The model under review builds one solid part; all positions refer to its coordinate system, in mm. Face numbers are marked on the shaded views. Give positions to 0.01 mm unless a question says otherwise; leave off trailing zeros. Loops run counter-clockwise (first coordinate to the right, second up) from the corner with the lowest first, then second, coordinate; pieces in that order, holes last. Notation, with made-up numbers: M 48,0.25 L 97,0.25 A25 ccw 97,35.25 Z; hole C -23.5,-16 d6. An arc over 180 degrees is marked long. One line per item, written item: value. Start each with the question number.
Q1. For pin 1 (3 mm diameter, centred on y = -3.11, z = 26.96, fed in from -X); pin 2 (1.5 mm diameter, centred on x = 0, y = 11, fed in from +Z); pin 3 (8 mm diameter, centred on x = -18.5, z = 3, fed in from -Y), all flat-tipped, find the tip position at first contact; note any pin that passes through.
Q2. Mouldability with a two-part tool opening along X and no side actions: class the marked faces 1, 2, 3 and 4 as released by +X, released by -X, zero draft, split by the parting line, or undercut.
Q3. We need section A-A on x = 0. Write out the cut boundary in (y, z).
Q4. We need section D-D on x = -11. Write out the cut boundary in (y, z).
Q5. To check wall thickness, follow line 1 along X through (y, z) = (-5, 15.5); line 2 along X through (y, z) = (0, -0.7); line 3 along Z through (x, y) = (-4, -10.5). State the ranges of each line that lie inside material, in increasing order. Write a range as from..to.
Q6. We need section B-B on z = 4.5. Write out the cut boundary in (x, y), plus the area to 3 significant figures.
Q7. We need section C-C on y = 11. Write out the cut boundary in (x, z), plus the area to 3 significant figures.
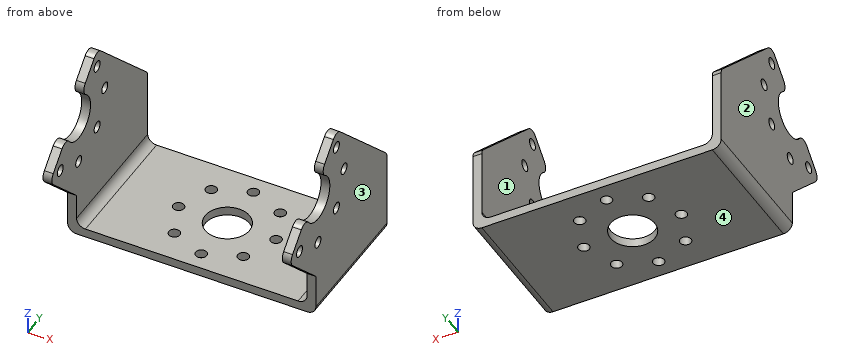
```python
from build123d import *

# Parameters (mm, degrees)
ESBO_O1_W                 = 56
ESBO_O1_H                 = 30
RESSALTO_EXTRUS_O1_DEPTH  = 2
RESSALTO_EXTRUS_O2_DEPTH  = 2
ESBO_O3_R                 = 5
CORTE_EXTRUS_O1_DEPTH     = 2
FILETE1_R                 = 2
ESBO_O4_R                 = 1.25
CORTE_EXTRUS_O2_DEPTH     = 2
PADR_OCIRCULAR1_COUNT     = 5
PADR_OCIRCULAR1_ANGLE     = 180
ESPELHAR3_COPY_1_SKETCH_R = 1.25
ESPELHAR3_COPY_1_DEPTH    = 2
ESPELHAR3_COPY_2_SKETCH_R = 1.25
ESPELHAR3_COPY_2_DEPTH    = 2
ESPELHAR3_COPY_3_SKETCH_R = 1.25
ESPELHAR3_COPY_3_DEPTH    = 2
ESPELHAR3_COPY_4_SKETCH_R = 1.25
ESPELHAR3_COPY_4_DEPTH    = 2
FILETE1_OF_ESPELHAR3_R    = 2
FILETE3_R                 = 2
ESBO_O5_R                 = 5
CORTE_EXTRUS_O3_DEPTH     = 2
ESBO_O6_R                 = 1.25
CORTE_EXTRUS_O4_DEPTH     = 2
PADR_OCIRCULAR2_COUNT     = 8


with BuildPart() as part:
    # Esboço1 → Ressalto-extrusão1 (new body)
    with BuildSketch(Plane.XY):
        Rectangle(ESBO_O1_W, ESBO_O1_H)
    extrude(amount=-RESSALTO_EXTRUS_O1_DEPTH)

    # Esboço2 → Ressalto-extrusão2 (add)
    with BuildSketch(Plane(origin=(28, 0, 0), x_dir=(0, 0, -1), z_dir=(1, 0, 0))):
        with BuildLine():
            Line((0, 15), (-17.021572875, 15))
            ThreePointArc((-17.021572875, 15), (-17.78693974, 14.847759065), (-18.435786438, 14.414213562))
            Line((-18.435786438, 14.414213562), (-37.651095085, -4.801095085))
            ThreePointArc((-37.651095085, -4.801095085), (-38.236880968, -6.21381893), (-37.653200295, -7.627413862))
            Line((-37.653200295, -7.627413862), (-20.507208242, -24.82456756))
            ThreePointArc((-20.507208242, -24.82456756), (-19.092379188, -25.412461791), (-17.676675908, -24.826675908))
            Line((-17.676675908, -24.826675908), (-7.85, -15))
            Line((-7.85, -15), (0, -15))
            Line((0, -15), (0, 15))
        make_face()
    ressalto_extrus_o2 = extrude(amount=-RESSALTO_EXTRUS_O2_DEPTH)

    # Esboço3 → Corte-extrusão1 (cut)
    with BuildSketch(Plane(origin=(28, 0, 0), x_dir=(0, 0, -1), z_dir=(1, 0, 0))):
        with Locations((-26.955270066, -14.108290294)):
            Circle(ESBO_O3_R)
    corte_extrus_o1 = extrude(amount=-CORTE_EXTRUS_O1_DEPTH, mode=Mode.SUBTRACT)

    # Filete1
    filete1_edges = [part.edges().sort_by_distance(p)[0] for p in [
        (27, -19.05908566, 26.255537796),
        (27, -13.393810572, 31.903958653),
    ]]
    fillet(filete1_edges, radius=FILETE1_R)

    # Esboço4 → Corte-extrusão2 (cut)
    with BuildSketch(Plane(origin=(28, 0, 0), x_dir=(0, 0, -1), z_dir=(1, 0, 0))):
        with Locations((-34.733444659, -6.330115701)):
            Circle(ESBO_O4_R)
    corte_extrus_o2 = extrude(amount=-CORTE_EXTRUS_O2_DEPTH, mode=Mode.SUBTRACT)

    # PadrãoCircular1: Corte-extrusão2 ×5 about axis
    padr_ocircular1_axis = Axis((0, -14.108290294, 26.955270066), (-1, 0, 0))
    for i in range(1, PADR_OCIRCULAR1_COUNT):
        add(corte_extrus_o2.rotate(padr_ocircular1_axis, i * PADR_OCIRCULAR1_ANGLE / (PADR_OCIRCULAR1_COUNT - 1)), mode=Mode.SUBTRACT)

    # Espelhar3: Ressalto-extrusão2, Corte-extrusão1, Corte-extrusão2 across plane
    add(ressalto_extrus_o2.mirror(Plane(origin=(0, 0, 0), x_dir=(0, 0, 1), z_dir=(1, 0, 0))))
    add(corte_extrus_o1.mirror(Plane(origin=(0, 0, 0), x_dir=(0, 0, 1), z_dir=(1, 0, 0))), mode=Mode.SUBTRACT)
    add(corte_extrus_o2.mirror(Plane(origin=(0, 0, 0), x_dir=(0, 0, 1), z_dir=(1, 0, 0))), mode=Mode.SUBTRACT)

    # Espelhar3 copy 1 sketch → Espelhar3 copy 1 (cut)
    with BuildSketch(Plane(origin=(-28, -23.192476809, -2.081051924), x_dir=(0, -0.7071067811865488, -0.7071067811865462), z_dir=(-1, 0, 0))):
        with Locations((-34.733444659, 6.330115701)):
            Circle(ESPELHAR3_COPY_1_SKETCH_R)
    extrude(amount=-ESPELHAR3_COPY_1_DEPTH, mode=Mode.SUBTRACT)

    # Espelhar3 copy 2 sketch → Espelhar3 copy 2 (cut)
    with BuildSketch(Plane(origin=(-28, -41.063560361, 12.846979772), x_dir=(0, -1, 0), z_dir=(-1, 0, 0))):
        with Locations((-34.733444659, 6.330115701)):
            Circle(ESPELHAR3_COPY_2_SKETCH_R)
    extrude(amount=-ESPELHAR3_COPY_2_DEPTH, mode=Mode.SUBTRACT)

    # Espelhar3 copy 3 sketch → Espelhar3 copy 3 (cut)
    with BuildSketch(Plane(origin=(-28, -43.144612285, 36.039456581), x_dir=(0, -0.7071067811865441, 0.7071067811865509), z_dir=(-1, 0, 0))):
        with Locations((-34.733444659, 6.330115701)):
            Circle(ESPELHAR3_COPY_3_SKETCH_R)
    extrude(amount=-ESPELHAR3_COPY_3_DEPTH, mode=Mode.SUBTRACT)

    # Espelhar3 copy 4 sketch → Espelhar3 copy 4 (cut)
    with BuildSketch(Plane(origin=(-28, -28.216580589, 53.910540133), x_dir=(0, 0, 1), z_dir=(-1, 0, 0))):
        with Locations((-34.733444659, 6.330115701)):
            Circle(ESPELHAR3_COPY_4_SKETCH_R)
    extrude(amount=-ESPELHAR3_COPY_4_DEPTH, mode=Mode.SUBTRACT)

    # Filete1 of Espelhar3
    filete1_of_espelhar3_edges = [part.edges().sort_by_distance(p)[0] for p in [
        (-27, -19.05908566, 26.255537796),
        (-27, -13.393810572, 31.903958653),
    ]]
    fillet(filete1_of_espelhar3_edges, radius=FILETE1_OF_ESPELHAR3_R)

    # Filete3
    filete3_edges = [part.edges().sort_by_distance(p)[0] for p in [
        (-28, 0, -2),
        (26, 0, 0),
        (28, 0, -2),
        (-26, 0, 0),
    ]]
    fillet(filete3_edges, radius=FILETE3_R)

    # Esboço5 → Corte-extrusão3 (cut)
    with BuildSketch(Plane.XY):
        Circle(ESBO_O5_R)
    corte_extrus_o3 = extrude(amount=-CORTE_EXTRUS_O3_DEPTH, mode=Mode.SUBTRACT)

    # Esboço6 → Corte-extrusão4 (cut)
    with BuildSketch(Plane.XY):
        with Locations((0, 11)):
            Circle(ESBO_O6_R)
    corte_extrus_o4 = extrude(amount=-CORTE_EXTRUS_O4_DEPTH, mode=Mode.SUBTRACT)

    # PadrãoCircular2: Corte-extrusão3, Corte-extrusão4 ×8 about axis
    padr_ocircular2_axis = Axis((0, 0, 0), (0, 0, 1))
    add([corte_extrus_o3.rotate(padr_ocircular2_axis, i * 360 / PADR_OCIRCULAR2_COUNT) for i in range(1, PADR_OCIRCULAR2_COUNT)], mode=Mode.SUBTRACT)
    add([corte_extrus_o4.rotate(padr_ocircular2_axis, i * 360 / PADR_OCIRCULAR2_COUNT) for i in range(1, PADR_OCIRCULAR2_COUNT)], mode=Mode.SUBTRACT)


solid = part.part
```
Solved:
1. pin 1: x = -28
1. pin 2: through
1. pin 3: y = -15
2. face 1: undercut
2. face 2: released by -X
2. face 3: released by +X
2. face 4: zero draft
3. outline: M -15,-2 L -12.25,-2 L -12.25,0 L -15,0 Z; M -9.75,-2 L -5,-2 L -5,0 L -9.75,0 Z; M 5,-2 L 9.75,-2 L 9.75,0 L 5,0 Z; M 12.25,-2 L 15,-2 L 15,0 L 12.25,0 Z
4. outline: M -15,-2 L -1.25,-2 L -1.25,0 L -15,0 Z; M 1.25,-2 L 15,-2 L 15,0 L 1.25,0 Z
5. line 1: -28..-26, 26..28
5. line 2: -27.87..-12.25, -9.75..-5, 5..9.75, 12.25..27.87
5. line 3: -2..0
6. outline: M -28,-15 L -26,-15 L -26,15 L -28,15 Z; M 26,-15 L 28,-15 L 28,15 L 26,15 Z
6. area: 120 mm2
7. outline: M -28,0 A2 ccw -26,-2 L -1.25,-2 L -1.25,0 L -24,0 A2 cw -26,2 L -26,21.85 L -28,21.85 Z; M 1.25,-2 L 26,-2 A2 ccw 28,0 L 28,21.85 L 26,21.85 L 26,2 A2 cw 24,0 L 1.25,0 Z
7. area: 194 mm2
